```python
from build123d import *

# Parameters (mm, degrees)
SKETCH1_W           = 48.26
SKETCH1_H           = 25.4
BOSS_EXTRUDE1_DEPTH = 6.35
SKETCH2_R           = 4.826
CUT_EXTRUDE1_DEPTH  = 8.89


with BuildPart() as part:
    # Sketch1 → Boss-Extrude1 (new body)
    with BuildSketch(Plane(origin=(0, 0, 0), x_dir=(1, 0, 0), z_dir=(0, 1, 0))):
        Rectangle(SKETCH1_W, SKETCH1_H)
    extrude(amount=BOSS_EXTRUDE1_DEPTH)

    # Sketch2 → Cut-Extrude1 (cut)
    with BuildSketch(Plane(origin=(0, 6.35, 0), x_dir=(1, 0, 0), z_dir=(0, 1, 0))):
        with Locations((-16.51, 0)):
            Circle(SKETCH2_R)
    extrude(amount=-CUT_EXTRUDE1_DEPTH, mode=Mode.SUBTRACT)


solid = part.part
```
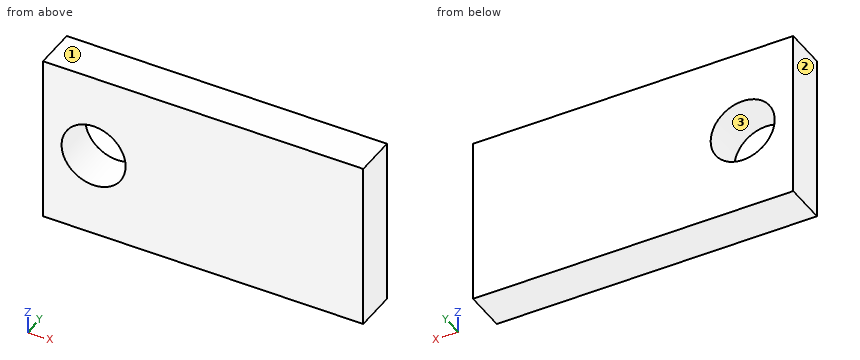
Could you check a few things on this model? Use its own coordinates, in mm. Face numbers are marked on the shaded views. Coordinates: 2 decimals unless noted, no trailing zeros. Write each loop counter-clockwise with the first axis right and the second up, starting at its lowest first coordinate (ties: lowest second). Pieces come first, ordered by that corner, then holes. Notation, with made-up numbers: (-9, -21) -> (23, -21) arc R19 ccw to (23, -16) -> close; hole circle Ø11 at (67, 36). An arc over 180 degrees is marked (long way). Write item = value, one per line. Start each with the question number.
(1) I want a section at B-B (x = -16.51). Please give me the cut outline in (y, z), plus the area to 4 significant figures.
(2) I want a section at A-A (z = 0). Please give me the cut outline in (x, y), plus the area to 3 significant figures.
(3) I want a section at C-C (y = 2.5). Please give me the cut outline in (x, z), plus the area to 3 significant figures.
(4) I need wall thicknesses on line 1 (Z direction, x = -16.51, y = 4.25); line 2 (X direction, y = 1.75, z = 0); line 3 (Z direction, x = -20.5, y = 3.5). Which ranges of each line are inside material? Lowest first, please. Write a range as [from, to].
(5) We'd pull the mould along Z, two halves only. Please class the marked faces 1, 2 and 3: released by +Z, released by -Z, zero draft, split by the parting line, or undercut.
Result set:
q1.outline = (0, -12.7) -> (6.35, -12.7) -> (6.35, -4.83) -> (0, -4.83) -> close; (0, 4.83) -> (6.35, 4.83) -> (6.35, 12.7) -> (0, 12.7) -> close
q1.area = 100.0 mm2
q2.outline = (-24.13, 0) -> (-21.34, 0) -> (-21.34, 6.35) -> (-24.13, 6.35) -> close; (-11.68, 0) -> (24.13, 0) -> (24.13, 6.35) -> (-11.68, 6.35) -> close
q2.area = 245 mm2
q3.outline = (-24.13, -12.7) -> (24.13, -12.7) -> (24.13, 12.7) -> (-24.13, 12.7) -> close; hole circle Ø9.65 at (-16.51, 0)
q3.area = 1,150 mm2
q4.line_1 = [-12.7, -4.83], [4.83, 12.7]
q4.line_2 = [-24.13, -21.34], [-11.68, 24.13]
q4.line_3 = [-12.7, -2.71], [2.71, 12.7]
q5.face_1 = released by +Z
q5.face_2 = zero draft
q5.face_3 = undercut
